```python
from build123d import *

# Parameters (mm, degrees)
IZIM1_R                     = 14
Y_KSEKLIK_EKSTR_ZYON1_DEPTH = 3
IZIM2_R                     = 7
Y_KSEKLIK_EKSTR_ZYON2_DEPTH = 15
IZIM3_R                     = 3
KES_EKSTR_ZYON1_DEPTH       = 18
IZIM4_R                     = 1.425
KES_EKSTR_ZYON2_DEPTH       = 18
DAIRESEL_KAPLAMA1_COUNT     = 4


with BuildPart() as part:
    # Çizim1 → Yükseklik-Ekstrüzyon1 (new body)
    with BuildSketch(Plane.XY):
        with Locations((-21.416051853, 15.917841079)):
            Circle(IZIM1_R)
    extrude(amount=Y_KSEKLIK_EKSTR_ZYON1_DEPTH)

    # Çizim2 → Yükseklik-Ekstrüzyon2 (add)
    with BuildSketch(Plane.XY.offset(3)):
        with Locations((-21.416051853, 15.917841079)):
            Circle(IZIM2_R)
    extrude(amount=Y_KSEKLIK_EKSTR_ZYON2_DEPTH)

    # Çizim3 → Kes-Ekstrüzyon1 (cut)
    with BuildSketch(Plane.XY.offset(18)):
        with Locations((-21.416051853, 15.917841079)):
            Circle(IZIM3_R)
    extrude(amount=-KES_EKSTR_ZYON1_DEPTH, mode=Mode.SUBTRACT)

    # Çizim4 → Kes-Ekstrüzyon2 (cut)
    with BuildSketch(Plane.XY.offset(3)):
        with Locations((-30.900018725, 15.917841079)):
            Circle(IZIM4_R)
    kes_ekstr_zyon2 = extrude(amount=-KES_EKSTR_ZYON2_DEPTH, mode=Mode.SUBTRACT)

    # Dairesel Kaplama1: Kes-Ekstrüzyon2 ×4 about axis
    dairesel_kaplama1_axis = Axis((-21.416051853, 15.917841079, 0), (0, 0, 1))
    for i in range(1, DAIRESEL_KAPLAMA1_COUNT):
        add(kes_ekstr_zyon2.rotate(dairesel_kaplama1_axis, i * 360 / DAIRESEL_KAPLAMA1_COUNT), mode=Mode.SUBTRACT)


solid = part.part
```
Can you work these out from the model? Positions are in its coordinate system, mm. A direction names the side the tool comes from. Give positions to 0.01 mm unless a question says otherwise; leave off trailing zeros. Loops run counter-clockwise (first coordinate to the right, second up) from the corner with the lowest first, then second, coordinate; pieces in that order, holes last. Notation, with made-up numbers: M 14.5,74.5 L 61.5,74.5 A12 cw 61.5,78.5 Z; hole C 50.25,16.5 d5. An arc over 180 degrees is marked long. Answer in a Markdown table with one row per item.
1. Suppose I cut it at C-C on z = 1.75. Write out the boundary of the cut face in (x, y) (3 decimals).
Taken from the geometry:
| item | result |
|---|---|
| outline | C -21.416,15.918 d28; hole C -30.9,15.918 d2.85; hole C -21.416,15.918 d6; hole C -21.416,6.434 d2.85; hole C -21.416,25.402 d2.85; hole C -11.932,15.918 d2.85 |
2. Suppose I cut it at D-D on x = -15.25. Write out the boundary of the cut face in (y, z), plus the area to 3 significant figures.
Taken from the geometry:
| item | result |
|---|---|
| outline | M 3.35,0 L 28.49,0 L 28.49,3 L 19.23,3 L 19.23,18 L 12.6,18 L 12.6,3 L 3.35,3 Z |
| area | 175 mm² |
3. If I drill on line 1 along Z through (x, y) = (-18.25, 27); line 2 along X through (y, z) = (26, 2.5); line 3 along X through (y, z) = (16.5, 14), over which ranges is the centre line in solid material (lowest first)?
Taken from the geometry:
| item | result |
|---|---|
| line 1 | z = 0 to 3 |
| line 2 | x = -31.13 to -22.71, -20.12 to -11.7 |
| line 3 | x = -28.39 to -24.36, -18.47 to -14.44 |
4. For pin 1 Ø8 at (y, z) = (17, 9.5) entering from +X; pin 2 Ø8 at (x, z) = (-30, 5.5) entering from -Y; pin 3 Ø2 at (y, z) = (11, 12) entering from -X, each with a flat end and sliding along its axis, tell me the tip position at first contact or that it passes through.
Taken from the geometry:
| item | result |
|---|---|
| pin 1 | stops at x = -14.42 |
| pin 2 | stops at y = 3.03 |
| pin 3 | stops at x = -27.22 |
5. Suppose I cut it at B-B on x = -31.25. Write out the boundary of the cut face in (y, z).
Taken from the geometry:
| item | result |
|---|---|
| outline | M 5.95,0 L 14.54,0 L 14.54,3 L 5.95,3 Z; M 17.3,0 L 25.88,0 L 25.88,3 L 17.3,3 Z |
6. Which directions (+Z, -Z, +X, -X, +Y, -Y) give clear straight access to the entire face, cutting with the end or side of a thin tool? Please do faces 1 (the cylindrical face through (-22.618, 7.2, 1.521)), 2 (the cylindrical face through (-26.97, 11.66, 10.4)).
Taken from the geometry:
| item | result |
|---|---|
| face 1 | +Z, -Z |
| face 2 | +Z |
7. Suppose I cut it at A-A on y = 17.75. Write out the boundary of the cut face in (x, z).
Taken from the geometry:
| item | result |
|---|---|
| outline | M -35.3,0 L -23.79,0 L -23.79,18 L -28.17,18 L -28.17,3 L -35.3,3 Z; M -19.04,0 L -7.54,0 L -7.54,3 L -14.66,3 L -14.66,18 L -19.04,18 Z |
8. Thinking about a two-plate mould opening in X: for faces 3 (the cylindrical face through (-23.627, 17.945, 9.126)), 4 (the cylindrical face through (-32.03, 15.05, 1.52)), 5 (the cylindrical face through (-8.48, 10.56, 1.48)), 6 (the flat face through (-18, 16, 18)), which applies, released by +X, released by -X, zero draft, split by the parting line, or undercut?
Taken from the geometry:
| item | result |
|---|---|
| face 3 | undercut |
| face 4 | undercut |
| face 5 | split by the parting line |
| face 6 | zero draft |
